```python
from build123d import *
from OCP.BRepFilletAPI import BRepFilletAPI_MakeChamfer

# Parameters (mm, degrees)
SKETCH1_R           = 2.5
SKETCH1_R_2         = 1.5
BOSS_EXTRUDE1_DEPTH = 10
CHAMFER1_SIZE       = 0.1
CHAMFER1_SIZE2      = 0.173205081


with BuildPart() as part:
    # Sketch1 → Boss-Extrude1 (new, symmetric)
    with BuildSketch(Plane.XY):
        Circle(SKETCH1_R)
        Circle(SKETCH1_R_2, mode=Mode.SUBTRACT)
    extrude(amount=BOSS_EXTRUDE1_DEPTH, both=True)

    # Chamfer1: one chamfer whose edges measure the first distance from different faces: ONE call of the kernel's chamfer builder (chamfer() names one face for all edges)
    chamfer1_edges_1 = [part.edges().sort_by_distance(p)[0] for p in [
        (-2.5, 0, -10),
    ]]
    chamfer1_side_1 = [part.faces().sort_by_distance(p)[0] for p in [
        (-2.429289322, 0, -10),
    ]]
    chamfer1_edges_2 = [part.edges().sort_by_distance(p)[0] for p in [
        (-2.5, 0, 10),
    ]]
    chamfer1_side_2 = [part.faces().sort_by_distance(p)[0] for p in [
        (-2.5, 0, 0),
    ]]
    chamfer1_edges_3 = [part.edges().sort_by_distance(p)[0] for p in [
        (-1.5, 0, -10),
    ]]
    chamfer1_side_3 = [part.faces().sort_by_distance(p)[0] for p in [
        (-1.5, 0, 0),
    ]]
    chamfer1_edges_4 = [part.edges().sort_by_distance(p)[0] for p in [
        (-1.5, 0, 10),
    ]]
    chamfer1_side_4 = [part.faces().sort_by_distance(p)[0] for p in [
        (-2.429289322, 0, 10),
    ]]
    chamfer1 = BRepFilletAPI_MakeChamfer(part.part.solid().wrapped)
    for e in chamfer1_edges_1:
        chamfer1.Add(CHAMFER1_SIZE, CHAMFER1_SIZE2, e.wrapped, chamfer1_side_1[0].wrapped)  # the first distance lies on this face
    for e in chamfer1_edges_2:
        chamfer1.Add(CHAMFER1_SIZE, CHAMFER1_SIZE2, e.wrapped, chamfer1_side_2[0].wrapped)  # the first distance lies on this face
    for e in chamfer1_edges_3:
        chamfer1.Add(CHAMFER1_SIZE, CHAMFER1_SIZE2, e.wrapped, chamfer1_side_3[0].wrapped)  # the first distance lies on this face
    for e in chamfer1_edges_4:
        chamfer1.Add(CHAMFER1_SIZE, CHAMFER1_SIZE2, e.wrapped, chamfer1_side_4[0].wrapped)  # the first distance lies on this face
    add(Compound.cast(chamfer1.Shape()), mode=Mode.REPLACE)


solid = part.part
```
Source: CAD feature listing. Evaluate the final solid. Frame: model axes, mm. Round coordinates to 2 decimals unless told otherwise and drop trailing zeros. Loops run counter-clockwise (first coordinate to the right, second up) from the corner with the lowest first, then second, coordinate; pieces in that order, holes last. Notation, with made-up numbers: (30.25, 74.25) - (44.25, 74.25) arc R37 cw to (44.25, 112.25) - close; hole circle Ø3 at (52.5, -34.5). An arc over 180 degrees is marked (long way). Use CSV: the item, a comma, the result in double quotes.
Q1. Ray query, line 1 along Y through (x, z) = (0.05, -2); line 2 along Y through (x, z) = (-1.15, 2); line 3 along X through (y, z) = (1.2, 5). Return the intervals inside material, ascending.
Reported:
line 1,"-2.5 to -1.5, 1.5 to 2.5"
line 2,"-2.22 to -0.96, 0.96 to 2.22"
line 3,"-2.19 to -0.9, 0.9 to 2.19"
Q2. Section query C-C, the plane z = -1. Output: boundary loops of the cut face in (x, y).
Reported:
outline,"circle Ø5 at (0, 0); hole circle Ø3 at (0, 0)"
Q3. Section query A-A, the plane x = 0. Output: boundary loops of the cut face in (y, z).
Reported:
outline,"(-2.5, -9.83) - (-2.4, -10) - (-1.67, -10) - (-1.5, -9.9) - (-1.5, 9.83) - (-1.6, 10) - (-2.33, 10) - (-2.5, 9.9) - close; (1.5, -9.9) - (1.67, -10) - (2.4, -10) - (2.5, -9.83) - (2.5, 9.9) - (2.33, 10) - (1.6, 10) - (1.5, 9.83) - close"
Q4. Pin query (flat end, axial travel): pin 1 Ø1 at (x, z) = (1, 0.5) entering from -Y; pin 2 Ø2 at (y, z) = (1, -7.5) entering from +X. Return the tip coordinate at first contact, or that it passes through.
Reported:
pin 1,"y = -2.45"
pin 2,"x = 2.5"
Q5. Mould query, pull axis X, two halves, no side actions, for faces 1 (the flat face through (-2, 0, -10)), 2 (the cylindrical face through (-0.54, -2.44, 0.17)), 3 (the cylindrical face through (-1.5, 0.07, -0.17)). Classes: pulls with the +X half, pulls with the -X half, needs draft (parallel to the pull), parting line crosses it, or undercut.
Reported:
face 1,"needs draft"
face 2,"parting line crosses it"
face 3,"undercut"
